Geometry check sheet. Reference: the model listing, model coordinates, mm. A direction names the side the tool comes from. Coordinates: 2 decimals unless noted, no trailing zeros. Write each loop counter-clockwise with the first axis right and the second up, starting at its lowest first coordinate (ties: lowest second). Pieces come first, ordered by that corner, then holes. Notation, with made-up numbers: M 11.5,74.25 L 44.5,74.25 A21 ccw 44.5,89.25 Z; hole C 62,65 d7. An arc over 180 degrees is marked long. Write each question's results on one line, items separated by ' | '.
```python
from build123d import *

# Parameters (mm, degrees)
F0_W     = 5
F0_H     = 5
F0_W_2   = 2.5
F0_H_2   = 10
F1_DEPTH = 5
F2_DEPTH = 7.5
F3_SIZE  = 2.49999


# Not quite as in the source:
# - a fillet or chamfer is up to 0.001 mm smaller than in the source, because OpenCascade refuses the exact size
# - a feature names something its author has since deleted; it is built from what else it names


with BuildPart() as f1:
    # F0 (on Top) → F1 (new body)
    with BuildSketch(Plane.XY):
        Polygon((-5, 5), (-2.5, 5), (2.5, 5), (5, 5), (7.5, 5), (25, 5), (25, 10), (-25, 10), (-25, 5), (-7.5, 5), align=None)
        Polygon((-57.5, 5), (-30, 5), (-30, 10), (-72.5, 10), (-72.5, 5), (-70, 5), (-67.5, 5), (-62.5, 5), (-60, 5), align=None)
        Polygon((-30, 10), (-25, 10), (-25, 47.5), (25, 47.5), (25, 10), (30, 10), (30, 52.5), (-30, 52.5), align=None)
        with Locations((-27.5, 7.5)):
            Rectangle(F0_W, F0_H)
        with Locations((-27.5, -7.5)):
            Rectangle(F0_W, F0_H)
        Polygon((-25, -47.5), (-25, -10), (-30, -10), (-30, -52.5), (30, -52.5), (30, -10), (25, -10), (25, -47.5), align=None)
        with Locations((27.5, 7.5)):
            Rectangle(F0_W, F0_H)
        Polygon((30, 10), (30, 5), (57.5, 5), (60, 5), (62.5, 5), (67.5, 5), (70, 5), (72.5, 5), (72.5, 10), align=None)
        with Locations((27.5, -7.5)):
            Rectangle(F0_W, F0_H)
        with Locations((61.25, 0)):
            Rectangle(F0_W_2, F0_H_2)
        with Locations((68.75, 0)):
            Rectangle(F0_W_2, F0_H_2)
        Polygon((2.5, -5), (-2.5, -5), (-5, -5), (-7.5, -5), (-25, -5), (-25, -10), (25, -10), (25, -5), (7.5, -5), (5, -5), align=None)
        with Locations((-3.75, 0)):
            Rectangle(F0_W_2, F0_H_2)
        with Locations((3.75, 0)):
            Rectangle(F0_W_2, F0_H_2)
        Polygon((-30, -10), (-30, -5), (-57.5, -5), (-60, -5), (-62.5, -5), (-67.5, -5), (-70, -5), (-72.5, -5), (-72.5, -10), align=None)
        with Locations((-68.75, 0)):
            Rectangle(F0_W_2, F0_H_2)
        with Locations((-61.25, 0)):
            Rectangle(F0_W_2, F0_H_2)
        with Locations((-71.25, 0)):
            Rectangle(F0_W_2, F0_H_2)
        with Locations((-58.75, 0)):
            Rectangle(F0_W_2, F0_H_2)
        Polygon((57.5, -5), (30, -5), (30, -10), (72.5, -10), (72.5, -5), (70, -5), (67.5, -5), (62.5, -5), (60, -5), align=None)
        with Locations((58.75, 0)):
            Rectangle(F0_W_2, F0_H_2)
        with Locations((71.25, 0)):
            Rectangle(F0_W_2, F0_H_2)
        with Locations((6.25, 0)):
            Rectangle(F0_W_2, F0_H_2)
        with Locations((-6.25, 0)):
            Rectangle(F0_W_2, F0_H_2)
        with Locations((-27.5, 0)):
            Rectangle(F0_W, F0_H_2)
        with Locations((27.5, 0)):
            Rectangle(F0_W, F0_H_2)
    extrude(amount=F1_DEPTH)

    # F0 (on Top) → F2 (join)
    with BuildSketch(Plane.XY):
        with Locations((-68.75, 0)):
            Rectangle(F0_W_2, F0_H_2)
        with Locations((-61.25, 0)):
            Rectangle(F0_W_2, F0_H_2)
        with Locations((-3.75, 0)):
            Rectangle(F0_W_2, F0_H_2)
        with Locations((3.75, 0)):
            Rectangle(F0_W_2, F0_H_2)
        with Locations((61.25, 0)):
            Rectangle(F0_W_2, F0_H_2)
        with Locations((68.75, 0)):
            Rectangle(F0_W_2, F0_H_2)
    extrude(amount=F2_DEPTH)

    # F3 (size 2.5 in the source; OpenCascade refuses exactly that, so slightly less here)
    f3_edges = [f1.edges().sort_by_distance(p)[0] for p in [
        (70, 0, 7.5),
        (60, 0, 7.5),
        (5, 0, 7.5),
        (-5, 0, 7.5),
        (-60, 0, 7.5),
        (-70, 0, 7.5),
    ]]
    chamfer(f3_edges, length=F3_SIZE)


solid = f1.part
```
Q1. Sectioned sample at D-D on y = 0. Give the number of separate pieces and of enclosed holes in the cut face, and give its area (3 significant figures).
Geometry check:
separate pieces: 8 | enclosed holes: 0 | area: 219 mm2
Q2. Scan lines: probe 1 along Y at (x, z) = (6, 2.25); probe 2 along Y at (x, z) = (1, 2.5); probe 3 along Y at (x, z) = (-38, 1.75). Record each from-to range of solid material in increasing order.
Geometry check:
probe 1: y = -52.5 to -47.5, -10 to 10, 47.5 to 52.5 | probe 2: y = -52.5 to -47.5, -10 to -5, 5 to 10, 47.5 to 52.5 | probe 3: y = -10 to -5, 5 to 10
Q3. Sectioned sample at A-A on y = -38.5. Record the cut outline in (x, z).
Geometry check:
outline: M -30,0 L -25,0 L -25,5 L -30,5 Z; M 25,0 L 30,0 L 30,5 L 25,5 Z
Q4. Access from +Z, -Z, +X, -X, +Y, -Y to the whole of each face (thin tool, end or side, straight path). Record for faces 1 (the flat face through (52, 10, 2)), 2 (the flat face through (25, 29, 2)).
Geometry check:
face 1: +Z, -Z, +X, +Y | face 2: +Z, -Z
Q5. Mould release check, pull along X, two halves, no side actions. Record for faces 3 (the flat face through (30, 31, 2)), 4 (the flat face through (-25, 0, 2)), 5 (the flat face through (-6, 0, 0)): pulls with the +X half, pulls with the -X half, needs draft (parallel to the pull), parting line crosses it, or undercut.
Geometry check:
face 3: pulls with the +X half | face 4: undercut | face 5: needs draft
Q6. Sectioned sample at B-B on x = 22.5. Record the cut outline in (y, z), and give its area (3 significant figures).
Geometry check:
outline: M -52.5,0 L -47.5,0 L -47.5,5 L -52.5,5 Z; M -10,0 L -5,0 L -5,5 L -10,5 Z; M 5,0 L 10,0 L 10,5 L 5,5 Z; M 47.5,0 L 52.5,0 L 52.5,5 L 47.5,5 Z | area: 100 mm2
Q7. Sectioned sample at C-C on x = 47. Record the cut outline in (y, z).
Geometry check:
outline: M -10,0 L -5,0 L -5,5 L -10,5 Z; M 5,0 L 10,0 L 10,5 L 5,5 Z
Q8. Depth check by flat-ended pin: P1, Ø4, axis at x = -64, z = 3.5, coming from the -Y side; P2, Ø4, axis at x = -64.5, z = 2.5, coming from the +Y side; P3, Ø0.8, axis at x = 69, z = 6.5, coming from the -Y side. Enter the tip coordinate at first touch or a pass-through.
Geometry check:
P1: stops at y = -10 | P2: stops at y = 10 | P3: stops at y = -5
